from build123d import *

# Parameters (mm, degrees)
F_6_CLEARANCE_HOLE1_D      = 3.7973
F_6_CLEARANCE_HOLE1_DEPTH  = 25.4
F_6_CLEARANCE_HOLE1_TIP    = 1.140824014
CUT_EXTRUDE1_DEPTH         = 128.563898106
F_6_CLEARANCE_HOLE2_D      = 3.7973
F_6_CLEARANCE_HOLE2_DEPTH  = 7.874
F_6_CLEARANCE_HOLE2_TIP    = 1.140824014
SKETCH11_R                 = 5.55625
BOSS_EXTRUDE1_DEPTH        = 9.525
CUT_EXTRUDE2_DEPTH         = 128.563898106
FILLET1_R                  = 9.525
M16X1_5_TAPPED_HOLE1_D     = 14.5
M16X1_5_TAPPED_HOLE1_DEPTH = 36.576
M16X1_5_TAPPED_HOLE1_TIP   = 4.356239488
F_6_32_TAPPED_HOLE2_D      = 2.7051
F_6_32_TAPPED_HOLE2_DEPTH  = 9.398
F_6_32_TAPPED_HOLE2_TIP    = 0.81269403


with BuildPart() as part:
    # Sketch1 → Revolve1 (revolve)
    with BuildSketch(Plane(origin=(0, 0, 0), x_dir=(1, 0, 0), z_dir=(0, 1, 0)), mode=Mode.PRIVATE) as revolve1_sk:
        Polygon((0, 0), (88.9, 0), (88.9, -6.35), (77.6478, -6.35), (77.6478, -3.7084), (73.025, -3.7084), (73.025, -6.35), (69.723, -6.35), (69.723, -11.176), (66.6242, -11.176), (66.6242, -15.113), (69.723, -15.113), (69.723, -18.288), (66.6242, -18.288), (66.6242, -22.225), (69.723, -22.225), (69.723, -25.4), (63.4492, -25.4), (63.4492, -3.81), (0, -3.81), align=None)
    revolve(revolve1_sk.sketch.rotate(Axis((0, 0, 0), (0, 0, 1)), 180), axis=Axis((0, 0, 0), (0, 0, 1)))

    # #6 Clearance Hole1
    with Locations(Plane.XY.offset(6.35)):
        with Locations((84.1375, 0), (25.999917364, -80.01951764), (-68.068667364, -49.454781665), (-68.068667364, 49.454781665), (25.999917364, 80.01951764)):
            Hole(F_6_CLEARANCE_HOLE1_D / 2, depth=F_6_CLEARANCE_HOLE1_DEPTH)
            with Locations((0, 0, -(F_6_CLEARANCE_HOLE1_DEPTH + F_6_CLEARANCE_HOLE1_TIP / 2))):  # 118° drill point
                Cone(0, F_6_CLEARANCE_HOLE1_D / 2, F_6_CLEARANCE_HOLE1_TIP, mode=Mode.SUBTRACT)

    # Sketch4 → Cut-Extrude1 (cut, through all)
    with BuildSketch(Plane.XY.offset(3.81)):
        with BuildLine():
            ThreePointArc((-11.7348, 26.5303), (-10.53144568, 27.02874568), (-10.033, 28.2321))
            Line((-10.033, 28.2321), (-10.033, 29.5275))
            ThreePointArc((-10.033, 29.5275), (-9.53455432, 30.73085432), (-8.3312, 31.2293))
            Line((-8.3312, 31.2293), (8.3312, 31.2293))
            ThreePointArc((8.3312, 31.2293), (9.53455432, 30.73085432), (10.033, 29.5275))
            Line((10.033, 29.5275), (10.033, 28.2321))
            ThreePointArc((10.033, 28.2321), (10.53144568, 27.02874568), (11.7348, 26.5303))
            Line((11.7348, 26.5303), (14.4272, 26.5303))
            Line((14.4272, 26.5303), (14.4272, 17.9197))
            Line((14.4272, 17.9197), (11.7348, 17.9197))
            ThreePointArc((11.7348, 17.9197), (10.53144568, 17.42125432), (10.033, 16.2179))
            Line((10.033, 16.2179), (10.033, 14.9225))
            ThreePointArc((10.033, 14.9225), (9.53455432, 13.71914568), (8.3312, 13.2207))
            Line((8.3312, 13.2207), (-8.3312, 13.2207))
            ThreePointArc((-8.3312, 13.2207), (-9.53455432, 13.71914568), (-10.033, 14.9225))
            Line((-10.033, 14.9225), (-10.033, 16.2179))
            ThreePointArc((-10.033, 16.2179), (-10.53144568, 17.42125432), (-11.7348, 17.9197))
            Line((-11.7348, 17.9197), (-14.4272, 17.9197))
            Line((-14.4272, 17.9197), (-14.4272, 26.5303))
            Line((-14.4272, 26.5303), (-11.7348, 26.5303))
        make_face()
        with BuildLine():
            Line((8.3312, 56.6293), (-8.3312, 56.6293))
            ThreePointArc((-8.3312, 56.6293), (-9.53455432, 56.13085432), (-10.033, 54.9275))
            Line((-10.033, 54.9275), (-10.033, 53.6321))
            ThreePointArc((-10.033, 53.6321), (-10.53144568, 52.42874568), (-11.7348, 51.9303))
            Line((-11.7348, 51.9303), (-14.4272, 51.9303))
            Line((-14.4272, 51.9303), (-14.4272, 43.3197))
            Line((-14.4272, 43.3197), (-11.7348, 43.3197))
            ThreePointArc((-11.7348, 43.3197), (-10.53144568, 42.82125432), (-10.033, 41.6179))
            Line((-10.033, 41.6179), (-10.033, 40.3225))
            ThreePointArc((-10.033, 40.3225), (-9.53455432, 39.11914568), (-8.3312, 38.6207))
            Line((-8.3312, 38.6207), (8.3312, 38.6207))
            ThreePointArc((8.3312, 38.6207), (9.53455432, 39.11914568), (10.033, 40.3225))
            Line((10.033, 40.3225), (10.033, 41.6179))
            ThreePointArc((10.033, 41.6179), (10.53144568, 42.82125432), (11.7348, 43.3197))
            Line((11.7348, 43.3197), (14.4272, 43.3197))
            Line((14.4272, 43.3197), (14.4272, 51.9303))
            Line((14.4272, 51.9303), (11.7348, 51.9303))
            ThreePointArc((11.7348, 51.9303), (10.53144568, 52.42874568), (10.033, 53.6321))
            Line((10.033, 53.6321), (10.033, 54.9275))
            ThreePointArc((10.033, 54.9275), (9.53455432, 56.13085432), (8.3312, 56.6293))
        make_face()
    extrude(amount=-CUT_EXTRUDE1_DEPTH, mode=Mode.SUBTRACT)

    # #6 Clearance Hole2
    with Locations(Plane.XY.offset(3.81)):
        with Locations((-18.4785, 47.625), (18.4785, 47.625), (-18.4785, 22.225), (18.4785, 22.225)):
            Hole(F_6_CLEARANCE_HOLE2_D / 2, depth=F_6_CLEARANCE_HOLE2_DEPTH)
            with Locations((0, 0, -(F_6_CLEARANCE_HOLE2_DEPTH + F_6_CLEARANCE_HOLE2_TIP / 2))):  # 118° drill point
                Cone(0, F_6_CLEARANCE_HOLE2_D / 2, F_6_CLEARANCE_HOLE2_TIP, mode=Mode.SUBTRACT)

    # Sketch11 → Boss-Extrude1 (add)
    with BuildSketch(Plane.XY.offset(3.81)):
        with BuildLine():
            Line((-48.930669698, 40.392951657), (-41.887522062, 34.040213285))
            ThreePointArc((-41.887522062, 34.040213285), (-42.094950568, 42.094950568), (-34.040213285, 41.887522062))
            Line((-34.040213285, 41.887522062), (-40.392951657, 48.930669698))
            ThreePointArc((-40.392951657, 48.930669698), (-44.865359581, 44.865359581), (-48.930669698, 40.392951657))
        make_face()
        with Locations((-38.166088515, 38.166088515)):
            Circle(SKETCH11_R)
        with Locations((38.166088515, 38.166088515)):
            Circle(SKETCH11_R)
        with BuildLine():
            ThreePointArc((43.722338515, 38.166088515), (43.242954143, 35.908357473), (41.887522062, 34.040213285))
            Line((41.887522062, 34.040213285), (48.930669698, 40.392951657))
            ThreePointArc((48.930669698, 40.392951657), (44.865359581, 44.865359581), (40.392951657, 48.930669698))
            Line((40.392951657, 48.930669698), (34.040213285, 41.887522062))
            ThreePointArc((34.040213285, 41.887522062), (40.159517698, 43.352431557), (43.722338515, 38.166088515))
        make_face()
        with Locations((38.166088515, -38.166088515)):
            Circle(SKETCH11_R)
        with BuildLine():
            Line((48.930669698, -40.392951657), (41.887522062, -34.040213285))
            ThreePointArc((41.887522062, -34.040213285), (43.242954143, -35.908357473), (43.722338515, -38.166088515))
            ThreePointArc((43.722338515, -38.166088515), (40.159517698, -43.352431557), (34.040213285, -41.887522062))
            Line((34.040213285, -41.887522062), (40.392951657, -48.930669698))
            ThreePointArc((40.392951657, -48.930669698), (44.865359581, -44.865359581), (48.930669698, -40.392951657))
        make_face()
        with BuildLine():
            ThreePointArc((-34.040213285, -41.887522062), (-42.094950568, -42.094950568), (-41.887522062, -34.040213285))
            Line((-41.887522062, -34.040213285), (-48.930669698, -40.392951657))
            ThreePointArc((-48.930669698, -40.392951657), (-44.865359581, -44.865359581), (-40.392951657, -48.930669698))
            Line((-40.392951657, -48.930669698), (-34.040213285, -41.887522062))
        make_face()
        with Locations((-38.166088515, -38.166088515)):
            Circle(SKETCH11_R)
    extrude(amount=BOSS_EXTRUDE1_DEPTH)

    # Sketch7 → Cut-Extrude2 (cut, through all)
    with BuildSketch(Plane.XY.offset(3.81)):
        with BuildLine():
            Line((52.761693969, -8.591783329), (49.988858988, -18.940144357))
            ThreePointArc((49.988858988, -18.940144357), (33.035725777, -8.851896043), (52.761693969, -8.591783329))
        make_face()
    extrude(amount=-CUT_EXTRUDE2_DEPTH, mode=Mode.SUBTRACT)

    # Fillet1
    # the kernel refuses this fillet: 9.525 mm, written as the material it adds along each edge
    with BuildSketch(Plane(origin=(-48.930669698, -40.392951657, 3.81), x_dir=(-0.5625955256004904, 0.8267322871246218, 0), z_dir=(0, 0, 1)), Plane(origin=(40.392951657, -48.930669698, 3.81), x_dir=(-0.8267322871246213, -0.5625955256004911, 0), z_dir=(0, 0, 1)), Plane(origin=(48.930669698, 40.392951657, 3.81), x_dir=(0.5625955256004896, -0.8267322871246222, 0), z_dir=(0, 0, 1)), Plane(origin=(-40.392951657, 48.930669698, 3.81), x_dir=(0.8267322871246212, 0.5625955256004912, 0), z_dir=(0, 0, 1))) as fillet1_piece_1:
        with BuildLine():
            CenterArc((10.85136124, -9.484206116), FILLET1_R, 84.695337095, 97.843486082)
            Line((1.335710636, -9.906128608), (0.384145576, -9.948320857))
            ThreePointArc((0.384145576, -9.948320857), (0.345915242, -9.526322078), (-0.943655336, -0.129502341))
            Line((-0.943655336, -0.129502341), (-0.08806017, 0.948420612))
            ThreePointArc((-0.08806017, 0.948420612), (5.865981471, 1.224241662), (11.820023112, 0.948420612))
            Line((11.820023112, 0.948420612), (11.731962942, 0))
        make_face()
    extrude(amount=9.525)
    with BuildSketch(Plane(origin=(-40.392951657, -48.930669698, 3.81), x_dir=(0.826732287124621, -0.5625955256004915, 0), z_dir=(0, 0, 1)), Plane(origin=(48.930669698, -40.392951657, 3.81), x_dir=(0.5625955256004891, 0.8267322871246228, 0), z_dir=(0, 0, 1)), Plane(origin=(40.392951657, 48.930669698, 3.81), x_dir=(-0.8267322871246218, 0.5625955256004905, 0), z_dir=(0, 0, 1)), Plane(origin=(-48.930669698, 40.392951657, 3.81), x_dir=(-0.5625955256004898, -0.8267322871246221, 0), z_dir=(0, 0, 1))) as fillet1_piece_2:
        with BuildLine():
            CenterArc((10.85136124, 9.484206116), FILLET1_R, 177.461176823, 97.843486082)
            Line((1.335710636, 9.906128608), (0.384145576, 9.948320857))
            ThreePointArc((0.384145576, 9.948320857), (0.345915242, 9.526322078), (-0.943655336, 0.129502341))
            Line((-0.943655336, 0.129502341), (-0.08806017, -0.948420612))
            ThreePointArc((-0.08806017, -0.948420612), (5.865981471, -1.224241662), (11.820023112, -0.948420612))
            Line((11.820023112, -0.948420612), (11.731962942, 0))
        make_face()
    extrude(amount=9.525)

    # M16x1.5 Tapped Hole1
    with Locations(Plane.XY.offset(3.81)):
        with Locations((44.752861065, 16.288709326), (-22.225, 0), (0, -22.225), (-16.288709326, -44.752861065), (-41.769336994, 15.202795371), (-41.769336994, -15.202795371), (16.288709326, -44.752861065)):
            Hole(M16X1_5_TAPPED_HOLE1_D / 2, depth=M16X1_5_TAPPED_HOLE1_DEPTH)
            with Locations((0, 0, -(M16X1_5_TAPPED_HOLE1_DEPTH + M16X1_5_TAPPED_HOLE1_TIP / 2))):  # 118° drill point
                Cone(0, M16X1_5_TAPPED_HOLE1_D / 2, M16X1_5_TAPPED_HOLE1_TIP, mode=Mode.SUBTRACT)

    # #6-32 Tapped Hole2
    with Locations(Plane.XY.offset(13.335)):
        with Locations((-38.166088515, 38.166088515), (38.166088515, 38.166088515), (38.166088515, -38.166088515), (-38.166088515, -38.166088515)):
            Hole(F_6_32_TAPPED_HOLE2_D / 2, depth=F_6_32_TAPPED_HOLE2_DEPTH)
            with Locations((0, 0, -(F_6_32_TAPPED_HOLE2_DEPTH + F_6_32_TAPPED_HOLE2_TIP / 2))):  # 118° drill point
                Cone(0, F_6_32_TAPPED_HOLE2_D / 2, F_6_32_TAPPED_HOLE2_TIP, mode=Mode.SUBTRACT)


solid = part.part
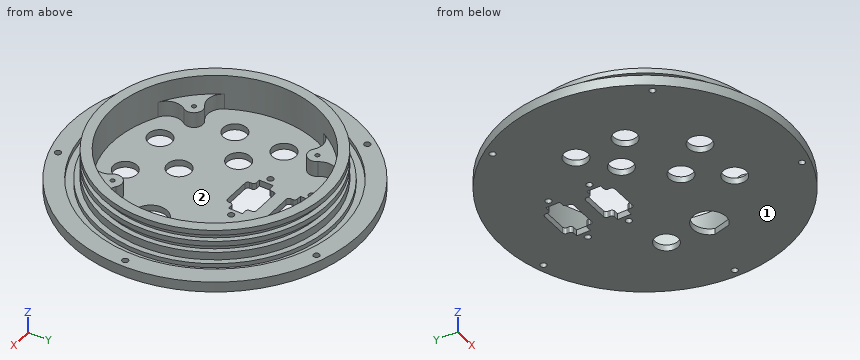
Geometry: final body of the model. Coordinates: model frame, mm. Face numbers are marked on the shaded views. A direction names the side the tool comes from. Round coordinates to 2 decimals unless told otherwise and drop trailing zeros.
Q1. Access query for the marked faces 1 and 2. Directions: +Z, -Z, +X, -X, +Y, -Y. A direction counts if a zero-diameter tool reaches every point of the face in a straight line with its end or side. Return the directions, or none.
Q2. Material intervals for L1, parallel to Z at x = -40, y = 56 (3 decimals); L2, parallel to X at y = 37.5, z = 9.25; L3, parallel to X at y = -49, z = 6.25, sorted ascending.
Q3. Pin query (flat end, axial travel): P1, Ø4, axis at x = -31.5, y = -11, coming from the +Z side; P2, Ø3, axis at x = -13.5, z = 2, coming from the +Y side; P3, Ø4, axis at y = 21.5, z = 2, coming from the +X side (3 decimals). Return the tip coordinate at first contact, or that it passes through.
Q4. Section A-A on x = 0. State how many separate pieces and enclosed holes the cut face has, plus the area to 3 significant figures.
Evaluation:
1. face 1: -Z, +X, -X, +Y, -Y
1. face 2: +Z
2. L1: z = 0 to 11.176, 15.113 to 18.288, 22.225 to 25.4
2. L2: x = -58.78 to -39.34, -36.99 to -32.65, 32.65 to 36.99, 39.34 to 58.78
2. L3: x = -74.18 to -69.91, -66.23 to -60.23, -54.14 to -35.44, 35.44 to 54.14, 60.23 to 74.18
3. P1: stops at z = 3.81
3. P2: stops at y = 88.09
3. P3: stops at x = 86.735
4. separate pieces: 4
4. enclosed holes: 0
4. area: 780 mm2
